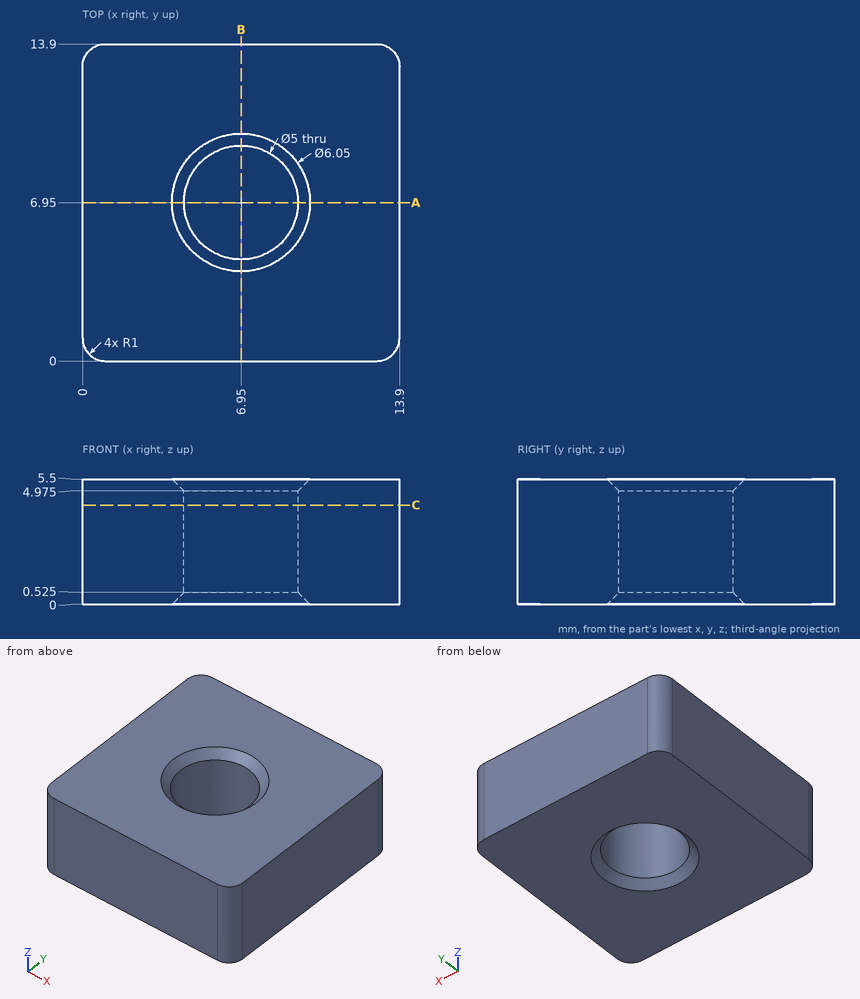
For this review, use the dimensioned drawing (mm, ordinates from the lowest corner) and the shaded views. Coordinates: 2 decimals unless noted, no trailing zeros. Loops run counter-clockwise (first coordinate to the right, second up) from the corner with the lowest first, then second, coordinate; pieces in that order, holes last. Notation, with made-up numbers: (1, -30.75) -> (28, -30.75) arc R30 cw to (28, 2.25) -> close; hole circle Ø10 at (0, 5.5). An arc over 180 degrees is marked (long way). Write each question's results on one line, items separated by ' | '.
Q1. To check wall thickness, follow line 1 along X through (y, z) = (6.95, 3.8); line 2 along Y through (x, z) = (8.5, 0.6). State the ranges of each line that lie inside material, in increasing order. Write a range as [from, to].
Taken from the geometry:
line 1: [0, 4.45], [9.45, 13.9] | line 2: [0, 4.99], [8.91, 13.9]
Q2. Add section C-C, the plane z = 4.35. State the section outline as (x, y) points, then the cut area to 3 significant figures.
Taken from the geometry:
outline: (0, 1) arc R1 ccw to (1, 0) -> (12.9, 0) arc R1 ccw to (13.9, 1) -> (13.9, 12.9) arc R1 ccw to (12.9, 13.9) -> (1, 13.9) arc R1 ccw to (0, 12.9) -> close; hole circle Ø5 at (6.95, 6.95) | area: 173 mm²
Q3. For pin 1 Ø4.5 at (x, y) = (6.95, 6.95) entering from -Z; pin 2 Ø1 at (x, z) = (5, 3) entering from -Y, all flat-tipped, find the tip position at first contact; note any pin that passes through.
Taken from the geometry:
pin 1: through | pin 2: y = 0
Q4. Add section A-A, the plane y = 6.95. State the section outline as (x, z) points (3 decimals), then the cut area to 3 significant figures.
Taken from the geometry:
outline: (0, 0) -> (3.925, 0) -> (4.45, 0.525) -> (4.45, 4.975) -> (3.925, 5.5) -> (0, 5.5) -> close; (9.45, 0.525) -> (9.975, 0) -> (13.9, 0) -> (13.9, 5.5) -> (9.975, 5.5) -> (9.45, 4.975) -> close | area: 48.4 mm²
